Check sheet for the drawn part. Datum: minimum x, y, z corner. Units: mm. A direction names the side the tool comes from. Round coordinates to 2 decimals unless told otherwise and drop trailing zeros. Write each loop counter-clockwise with the first axis right and the second up, starting at its lowest first coordinate (ties: lowest second). Pieces come first, ordered by that corner, then holes. Notation, with made-up numbers: (34, -19) -> (77, -19) arc R12 cw to (77, 3) -> close; hole circle Ø9 at (-34.5, 39). An arc over 180 degrees is marked (long way). One line per item, written item: value.
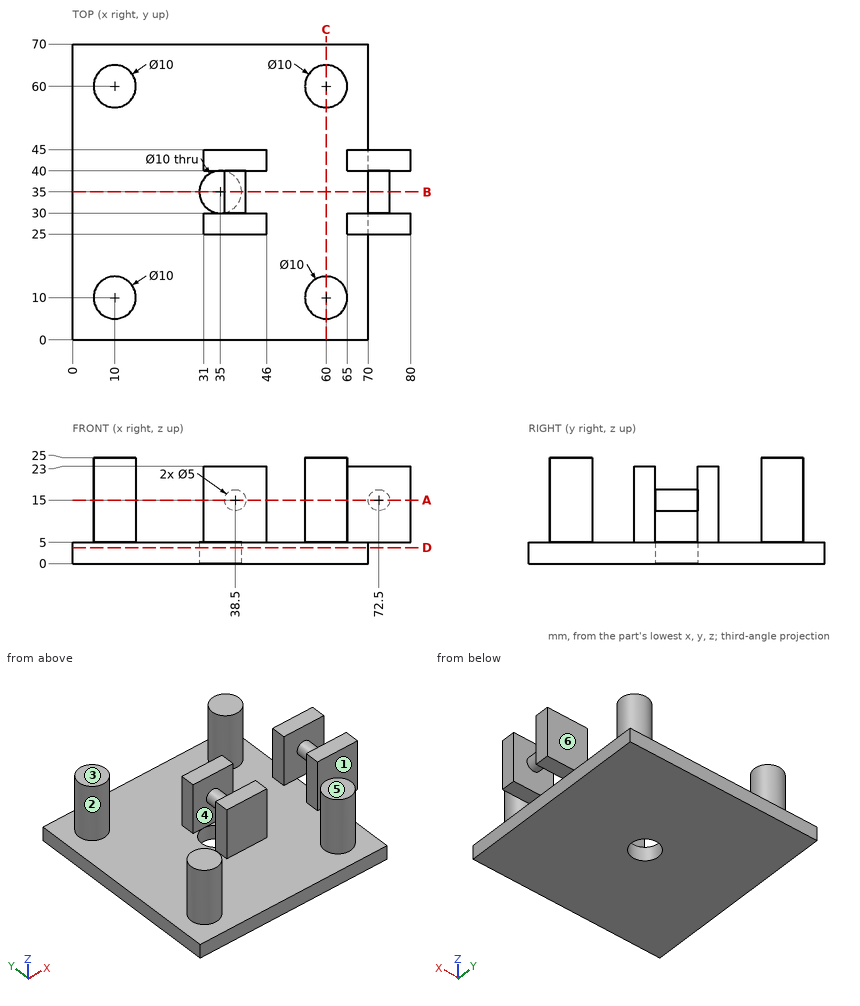
Item 1: Sectioned sample at D-D on z = 3.75. Enter the section's corners in (x, y).
Answer:
outline: (0, 0) -> (70, 0) -> (70, 70) -> (0, 70) -> close; hole circle Ø10 at (35, 35)
Item 2: Mould release check, pull along Z, two halves, no side actions. Record for the marked faces 4, 5 and 6: pulls with the +Z half, pulls with the -Z half, needs draft (parallel to the pull), parting line crosses it, or undercut.
Answer:
face 4: undercut
face 5: pulls with the +Z half
face 6: needs draft
Item 3: Sectioned sample at B-B on y = 35. Enter the section's corners in (x, z).
Answer:
outline: (0, 0) -> (30, 0) -> (30, 5) -> (0, 5) -> close; circle Ø5 at (38.5, 15); (40, 0) -> (70, 0) -> (70, 5) -> (40, 5) -> close; circle Ø5 at (72.5, 15)
Item 4: Depth check by flat-ended pin: P1, Ø6, axis at x = 25, y = 19, coming from the +Z side; P2, Ø1, axis at y = 27, z = 13.5, coming from the -X side; P3, Ø2.5, axis at x = 72.5, y = 42.5, coming from the -Z side; P4, Ø10, axis at x = 20.5, z = 20, coming from the -Y side. Enter the tip coordinate at first touch or a pass-through.
Answer:
P1: stops at z = 5
P2: stops at x = 31
P3: stops at z = 5
P4: passes through
Item 5: Sectioned sample at A-A on z = 15. Enter the section's corners in (x, y).
Answer:
outline: circle Ø10 at (10, 10); circle Ø10 at (10, 60); (31, 25) -> (46, 25) -> (46, 30) -> (41, 30) -> (41, 40) -> (46, 40) -> (46, 45) -> (31, 45) -> (31, 40) -> (36, 40) -> (36, 30) -> (31, 30) -> close; circle Ø10 at (60, 10); circle Ø10 at (60, 60); (65, 25) -> (80, 25) -> (80, 30) -> (75, 30) -> (75, 40) -> (80, 40) -> (80, 45) -> (65, 45) -> (65, 40) -> (70, 40) -> (70, 30) -> (65, 30) -> close
Item 6: Thickness scan on line 1 (X direction, y = 35, z = 1.2); line 2 (Y direction, x = 76, z = 17.25); line 3 (X direction, y = 43, z = 20.5). Record the ranges inside material, lowest first.
Answer:
line 1: x = 0 to 30, 40 to 70
line 2: y = 25 to 30, 40 to 45
line 3: x = 31 to 46, 65 to 80
Item 7: Sectioned sample at C-C on x = 60. Enter the section's corners in (y, z).
Answer:
outline: (0, 0) -> (70, 0) -> (70, 5) -> (65, 5) -> (65, 25) -> (55, 25) -> (55, 5) -> (15, 5) -> (15, 25) -> (5, 25) -> (5, 5) -> (0, 5) -> close
Item 8: Tool access check on the marked faces 1, 2 and 3. Record the directions out of +Z, -Z, +X, -X, +Y, -Y that give a thin tool (end or side, any length) a straight path to the whole face; none if there is none.
Answer:
face 1: +Z, +X, -X, -Y
face 2: +Z
face 3: +Z, +X, -X, +Y, -Y
